Could you check a few things on this drawing? It's one solid part, dimensions in mm from its lowest x, y, z. A direction names the side the tool comes from. Round coordinates to 2 decimals unless told otherwise and drop trailing zeros. Loops run counter-clockwise (first coordinate to the right, second up) from the corner with the lowest first, then second, coordinate; pieces in that order, holes last. Notation, with made-up numbers: M 51,70.5 L 95,70.5 A21 ccw 95,105.5 Z; hole C 79,31.25 d8. An arc over 180 degrees is marked long. Answer as CSV lines item,"result".
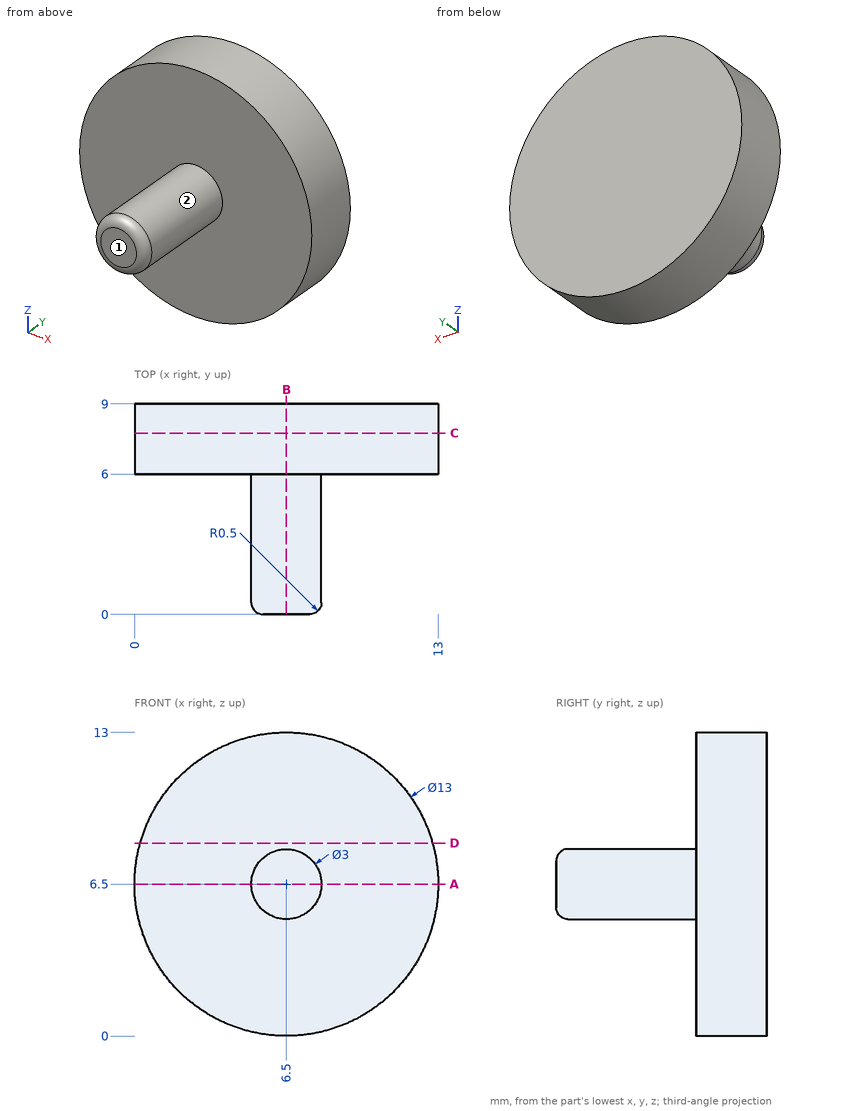
Item 1: If we section it at C-C on y = 7.75: Write out the boundary of the cut face in (x, z), then the cut area to 3 significant figures.
Output:
outline,"C 6.5,6.5 d13"
area,"133 mm2"
Item 2: On a 3-axis mill with a long thin cutter (end or side, diameter ignored), from which of +Z, -Z, +X, -X, +Y, -Y can I reach the whole of each face in a straight line? I mean the marked faces 1 and 2. Say none if no direction works.
Output:
face 1,"+Z, -Z, +X, -X, -Y"
face 2,"-Y"
Item 3: If we section it at B-B on x = 6.5: Write out the boundary of the cut face in (y, z), then the cut area to 3 significant figures.
Output:
outline,"M 0,5.5 A0.5 ccw 0.5,5 L 6,5 L 6,0 L 9,0 L 9,13 L 6,13 L 6,8 L 0.5,8 A0.5 ccw 0,7.5 Z"
area,"56.9 mm2"
Item 4: Will this pin go through, and if not, where does the flat tip stop? pin 1 (4 mm diameter, centred on y = 2.5, z = 8.5, fed in from +X).
Output:
pin 1,"stops at x = 8"
Item 5: If we section it at A-A on z = 6.5: Write out the boundary of the cut face in (x, y), then the cut area to 3 significant figures.
Output:
outline,"M 0,6 L 5,6 L 5,0.5 A0.5 ccw 5.5,0 L 7.5,0 A0.5 ccw 8,0.5 L 8,6 L 13,6 L 13,9 L 0,9 Z"
area,"56.9 mm2"
Item 6: If I drill on line 1 along Y through (x, z) = (1.5, 7); line 2 along Y through (x, z) = (7.5, 7); line 3 along Z through (x, y) = (10.25, 8.5), over which ranges is the centre line in solid material (lowest first)? Write a range as from..to.
Output:
line 1,"y = 6..9"
line 2,"y = 0.01..9"
line 3,"z = 1.19..11.81"
Item 7: If we section it at D-D on z = 8.25: Write out the boundary of the cut face in (x, y), then the cut area to 3 significant figures.
Output:
outline,"M 0.24,6 L 12.76,6 L 12.76,9 L 0.24,9 Z"
area,"37.6 mm2"
